```python
from build123d import *

# Parameters (mm, degrees)
SKETCH1_R           = 18.099999995
BOSS_EXTRUDE1_DEPTH = 33.3
SKETCH2_R           = 18.5
BOSS_EXTRUDE2_DEPTH = 24.5
SKETCH3_R           = 5.999999938
BOSS_EXTRUDE3_DEPTH = 5
SKETCH4_R           = 1.500000048
BOSS_EXTRUDE4_DEPTH = 15
CUT_EXTRUDE2_START  = -14
CUT_EXTRUDE2_DEPTH  = 14


with BuildPart() as part:
    # Sketch1 → Boss-Extrude1 (new body)
    with BuildSketch(Plane.XY):
        Circle(SKETCH1_R)
    extrude(amount=BOSS_EXTRUDE1_DEPTH)

    # Sketch2 → Boss-Extrude2 (add)
    with BuildSketch(Plane.XY.offset(33.3)):
        Circle(SKETCH2_R)
    extrude(amount=BOSS_EXTRUDE2_DEPTH)

    # Sketch3 → Boss-Extrude3 (add)
    with BuildSketch(Plane.XY.offset(57.8)):
        Circle(SKETCH3_R)
    extrude(amount=BOSS_EXTRUDE3_DEPTH)

    # Sketch4 → Boss-Extrude4 (add)
    with BuildSketch(Plane.XY.offset(62.8)):
        Circle(SKETCH4_R)
    extrude(amount=BOSS_EXTRUDE4_DEPTH)

    # Sketch8 → Cut-Extrude2 (cut)
    with BuildSketch(Plane.XY.offset(77.8).offset(CUT_EXTRUDE2_START)):
        with BuildLine():
            Line((-1.118034025, 1.000000032), (1.118034025, 1.000000032))
            ThreePointArc((1.118034025, 1.000000032), (0, 1.500000048), (-1.118034025, 1.000000032))
        make_face()
    extrude(amount=CUT_EXTRUDE2_DEPTH, mode=Mode.SUBTRACT)


solid = part.part
```
CAD build for the part. Positions are in the model's coordinates, mm. A direction names the side the tool comes from. Round coordinates to 2 decimals unless told otherwise and drop trailing zeros. Order: outer loops, then holes, each group sorted by start corner. A loop starts at its lowest first (then second) coordinate and runs counter-clockwise, first axis right, second up.
Q1. Slice it at D-D (x = 12). Write the cut outline in (y, z), and give its area (3 significant figures).
Q2. Drop flat-ended pins along their axis: pin 1 (3 mm diameter, centred on x = -7, z = 19.5, fed in from +Y); pin 2 (3 mm diameter, centred on x = 8.5, y = -1, fed in from +Z); pin 3 (6 mm diameter, centred on y = 6, z = 37, fed in from -X). Give the stop position or say it passes through.
Q3. Slice it at C-C (z = 29). Write the cut outline in (x, y).
Q4. Wall check: L1, parallel to Z at x = 10.5, y = -3; L2, parallel to Z at x = -1.5, y = 5; L3, parallel to X at y = -12.5, z = 27. Give the ranges that are in metal, low to high.
Q5. Which spindle directions (+Z, -Z, +X, -X, +Y, -Y) get a long thin tool onto all of the face, cutting with end or side? Do faces 1 (the cylindrical face through (-4.42, 4.06, 60.26)), 2 (the flat face through (0, 1, 71)), 3 (the flat face through (13.6, -12.2, 33.3)). Say none if no direction does.
Q6. Slice it at A-A (y = 0). Write the cut outline in (x, z).
Q7. Slice it at B-B (x = -16). Write the cut outline in (y, z).
Results below:
1. outline: (-14.08, 33.3) - (-13.55, 33.3) - (-13.55, 0) - (13.55, 0) - (13.55, 33.3) - (14.08, 33.3) - (14.08, 57.8) - (-14.08, 57.8) - close
1. area: 1,590 mm2
2. pin 1: stops at y = 17.24
2. pin 2: stops at z = 57.8
2. pin 3: stops at x = -18.26
3. outline: circle Ø36.2 at (0, 0)
4. L1: z = 0 to 57.8
4. L2: z = 0 to 62.8
4. L3: x = -13.09 to 13.09
5. face 1: +Z
5. face 2: +Z, +X, -X, +Y
5. face 3: -Z
6. outline: (-18.5, 33.3) - (-18.1, 33.3) - (-18.1, 0) - (18.1, 0) - (18.1, 33.3) - (18.5, 33.3) - (18.5, 57.8) - (6, 57.8) - (6, 62.8) - (1.5, 62.8) - (1.5, 77.8) - (-1.5, 77.8) - (-1.5, 62.8) - (-6, 62.8) - (-6, 57.8) - (-18.5, 57.8) - close
7. outline: (-9.29, 33.3) - (-8.46, 33.3) - (-8.46, 0) - (8.46, 0) - (8.46, 33.3) - (9.29, 33.3) - (9.29, 57.8) - (-9.29, 57.8) - close
